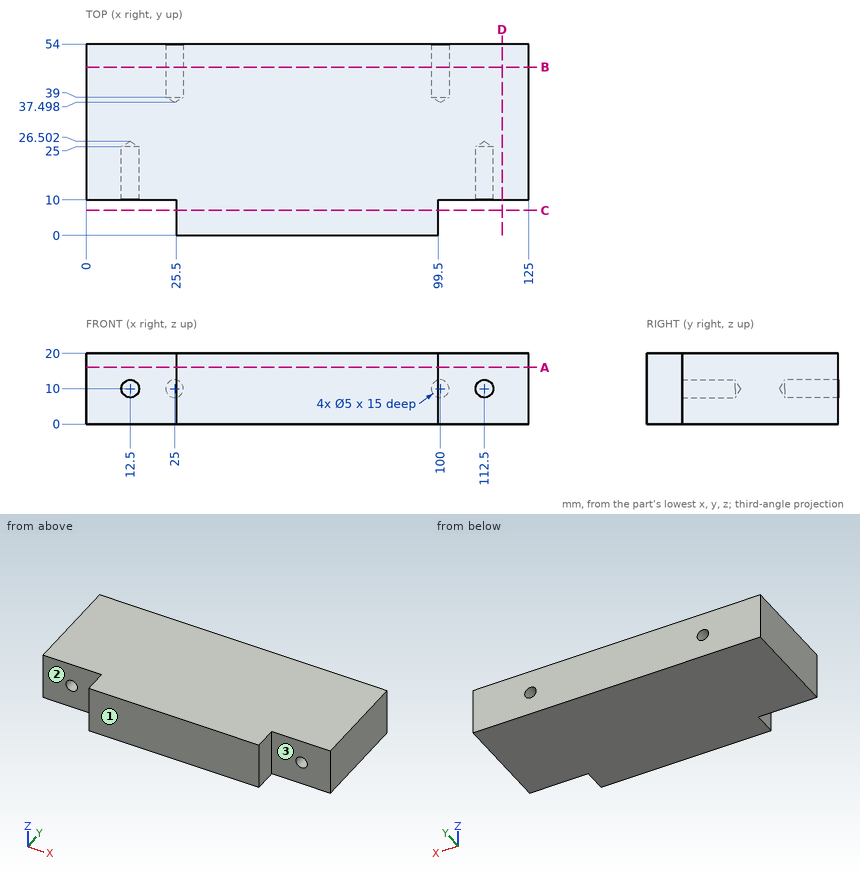
Could you check a few things on this drawing? It's one solid part, dimensions in mm from its lowest x, y, z. A direction names the side the tool comes from. Give positions to 0.01 mm unless a question says otherwise; leave off trailing zeros. Order: outer loops, then holes, each group sorted by start corner. A loop starts at its lowest first (then second) coordinate and runs counter-clockwise, first axis right, second up. Notation, with made-up numbers: (42, 80.5) - (64, 80.5) arc R26 cw to (64, 94.5) - close; hole circle Ø1 at (-35.75, -35.75). An arc over 180 degrees is marked (long way). One line per question, with ' | ' between items. Start each with the question number.
Item 1: I'm going to push flat-ended pins straight in: pin 1 Ø4 at (x, z) = (25, 10) entering from +Y; pin 2 Ø3 at (y, z) = (7.5, 3.5) entering from +X; pin 3 Ø6 at (x, z) = (12.5, 10) entering from -Y. Where does each tip first touch, or does it pass through?
Item 2: I want a section at D-D on x = 117.5. Write out the boundary of the cut face in (y, z), then the cut area to 3 significant figures.
Item 3: I want a section at B-B on y = 47.5. Write out the boundary of the cut face in (x, z), then the cut area to 3 significant figures.
Item 4: For the marked faces 1, 2 and 3, which set-ups out of +Z, -Z, +X, -X, +Y, -Y let a thin tool reach every point of the face, with its end or its side?
Item 5: I need wall thicknesses on probe 1 along X at (y, z) = (21, 10); probe 2 along X at (y, z) = (46.5, 10); probe 3 along Z at (x, y) = (25, 50.5). Which ranges of each line are inside material? Lowest first, please. Write a range as [from, to].
Item 6: I want a section at C-C on y = 7. Write out the boundary of the cut face in (x, z).
Item 7: I want a section at A-A on z = 16. Write out the boundary of the cut face in (x, y).
Verdict:
1) pin 1: y = 38.7 | pin 2: x = 99.5 | pin 3: y = 10
2) outline: (10, 0) - (54, 0) - (54, 20) - (10, 20) - close | area: 880 mm^2
3) outline: (0, 0) - (125, 0) - (125, 20) - (0, 20) - close; hole circle Ø5 at (25, 10); hole circle Ø5 at (100, 10) | area: 2,460 mm^2
4) face 1: +Z, -Z, +X, -X, -Y | face 2: +Z, -Z, -X, -Y | face 3: +Z, -Z, +X, -Y
5) probe 1: [0, 10], [15, 110], [115, 125] | probe 2: [0, 22.5], [27.5, 97.5], [102.5, 125] | probe 3: [0, 7.5], [12.5, 20]
6) outline: (25.5, 0) - (99.5, 0) - (99.5, 20) - (25.5, 20) - close
7) outline: (0, 10) - (25.5, 10) - (25.5, 0) - (99.5, 0) - (99.5, 10) - (125, 10) - (125, 54) - (0, 54) - close
